The model under review builds one solid part; all positions refer to its coordinate system, in mm. A direction names the side the tool comes from. Coordinates: 2 decimals unless noted, no trailing zeros. Loops run counter-clockwise (first coordinate to the right, second up) from the corner with the lowest first, then second, coordinate; pieces in that order, holes last. Notation, with made-up numbers: M -3,-40 L 39,-40 A19 cw 39,-22 Z; hole C 16.5,45 d3. An arc over 180 degrees is marked long. Use one line per item in the form item = value.
```python
from build123d import *

# Parameters (mm, degrees)
F1_ANGLE = 180
F2_DEPTH = 5.08
F0_W     = 3.2131851465
F0_H     = 5.0839147031
F0_H_2   = 5.0760852969
F0_W_2   = 5.092757754
F0_H_3   = 2.607280938
F3_DEPTH = 5.08


with BuildPart() as f1:
    # F0 (on Front) → F1 (revolve)
    with BuildSketch(Plane.XZ):
        with BuildLine():
            Line((0, 7.1843154948), (0, 9.2163154948))
            Line((0, 9.2163154948), (-5.092757754, 9.2163154948))
            Line((-5.092757754, 9.2163154948), (-12.192, 9.2163154948))
            ThreePointArc((-12.192, 9.2163154948), (-11.524233364, 1.2175235719), (-11.5414183138, -6.8090752834))
            Line((-11.5414183138, -6.8090752834), (-10.7442, -6.8090752834))
            Line((-10.7442, -6.8090752834), (-10.7442, -16.9690752834))
            Line((-10.7442, -16.9690752834), (-12.55264014, -16.9690752834))
            ThreePointArc((-12.55264014, -16.9690752834), (-14.3638496802, -25.8279076884), (-17.018, -34.4716845052))
            Line((-17.018, -34.4716845052), (-14.986, -34.4716845052))
            ThreePointArc((-14.986, -34.4716845052), (-9.9329646545, -13.9500940953), (-10.0076, 7.1843154948))
            Line((-10.0076, 7.1843154948), (0, 7.1843154948))
        make_face()
        with BuildLine():
            Line((-10.7442, -6.8090752834), (-11.5414183138, -6.8090752834))
            ThreePointArc((-11.5414183138, -6.8090752834), (-11.908955512, -11.9028177198), (-12.55264014, -16.9690752834))
            Line((-12.55264014, -16.9690752834), (-10.7442, -16.9690752834))
            Line((-10.7442, -16.9690752834), (-10.7442, -6.8090752834))
        make_face()
    revolve(axis=Axis((0, 0, 8.2003154948), (0, 0, -1)), revolution_arc=F1_ANGLE)

    # F0 (on Front) → F2 (join)
    with BuildSketch(Plane.XZ):
        with BuildLine():
            ThreePointArc((-12.55264014, -16.9690752834), (-11.908955512, -11.9028177198), (-11.5414183138, -6.8090752834))
            Line((-11.5414183138, -6.8090752834), (-12.55264014, -6.8090752834))
            Line((-12.55264014, -6.8090752834), (-12.55264014, -11.8851605803))
            Line((-12.55264014, -11.8851605803), (-12.55264014, -16.9690752834))
        make_face()
        with BuildLine():
            Line((-10.7442, -6.8090752834), (-11.5414183138, -6.8090752834))
            ThreePointArc((-11.5414183138, -6.8090752834), (-11.908955512, -11.9028177198), (-12.55264014, -16.9690752834))
            Line((-12.55264014, -16.9690752834), (-10.7442, -16.9690752834))
            Line((-10.7442, -16.9690752834), (-10.7442, -6.8090752834))
        make_face()
        Polygon((12.55264014, -6.9773710036), (10.7442, -6.9773710036), (10.7442, -17.1373710036), (12.55264014, -17.1373710036), (12.55264014, -12.0534563005), align=None)
    extrude(amount=-F2_DEPTH)

    # F0 (on Front) → F3 (join, symmetric)
    with BuildSketch(Plane.XZ):
        with Locations((14.1592327132, -14.5954136521)):
            Rectangle(F0_W, F0_H)
        with Locations((-14.1592327132, -9.3471179318)):
            Rectangle(F0_W, F0_H_2)
        with Locations((-2.546378877, 10.5199559638)):
            Rectangle(F0_W_2, F0_H_3)
    extrude(amount=F3_DEPTH, both=True)


solid = f1.part
```
1. Add section A-A (y = -2.75). State the section outline as (x, z) points, then the cut area to 3 significant figures.
Response values:
outline = M -15.77,-11.89 L -12.55,-11.89 L -12.55,-6.81 L -15.77,-6.81 Z; M -5.09,9.22 L 0,9.22 L 0,11.82 L -5.09,11.82 Z; M 12.55,-17.14 L 15.77,-17.14 L 15.77,-12.05 L 12.55,-12.05 Z
area = 45.9 mm^2
2. Add section B-B (z = -14). State the section outline as (x, y) points, then the cut area to 3 significant figures.
Response values:
outline = M -12.55,0 L -9.94,0 A9.94 cw 9.94,0 L 12.55,0 L 12.55,-5.08 L 15.77,-5.08 L 15.77,5.08 L 11.03,5.08 A12.14 ccw -11.03,5.08 L -12.55,5.08 Z
area = 117 mm^2
3. Machinability: for faces 5 (the face through (12.553, 3, -10)), 6 (the face through (-13, 5.08, -11)), 7 (the face through (13, 5.08, -13)), 8 (the face through (-3, 5.08, 11)), which of the approach directions +Z, -Z, +X, -X, +Y, -Y give a long, thin tool a straight path to every point of the face, cutting with its end or side? Answer none if there is none.
Response values:
face_5 = +Z, +X, +Y, -Y
face_6 = -X, +Y
face_7 = +X, +Y
face_8 = +Z, +X, -X, +Y
4. The part is to be moulded in two halves that separate along Z. For faces 1 (the face through (-14, 0, -11.885)), 2 (the face through (-12.553, -3, -9)), 3 (the face through (-12.553, 3, -14)), 4 (the face through (14, 0, -12.053)), say which applies: pulls with the +Z half, pulls with the -Z half, needs draft (parallel to the pull), parting line crosses it, or undercut.
Response values:
face_1 = undercut
face_2 = needs draft
face_3 = undercut
face_4 = pulls with the +Z half
5. Insertion check: P1, Ø1.5, axis at x = 3, z = -7.5, coming from the +Y side; P2, Ø1.5, axis at y = 12.5, z = -25.5, coming from the -X side; P3, Ø1, axis at x = 4.5, z = 0, coming from the +Y side; P4, Ø3.5, axis at x = 13.5, y = 0.5, coming from the -Z side. Each pin has a flat end and moves straight along its axis. Give the tip position at first contact, or say it passes through.
Response values:
P1 = 11.36
P2 = -8.17
P3 = 10.76
P4 = -34.47
6. Add section D-D (z = 0.5). State the section outline as (x, y) points, then the cut area to 3 significant figures.
Response values:
outline = M -11.5,0 L -9.42,0 A9.42 cw 9.42,0 L 11.5,0 A11.5 ccw Z
area = 68.2 mm^2
7. Add section C-C (z = -7.5). State the section outline as (x, y) points.
Response values:
outline = M -15.77,-5.08 L -12.55,-5.08 L -12.55,0 L -9.41,0 A9.41 cw 9.41,0 L 12.55,0 L 12.55,5.08 L 10.74,5.08 L 10.74,4.31 A11.57 ccw -10.74,4.31 L -10.74,5.08 L -15.77,5.08 Z
8. Wall thickness on line 1 along Z through (x, y) = (-8.5, 2.25); line 2 along X through (y, z) = (3, -16.5); line 3 along X through (y, z) = (-3.25, -10): over which ranges is each line inside the solid? List them lowest first. Write a range as from..to.
Response values:
line_1 = 7.18..9.22
line_2 = -12.55..-9.83, 9.83..15.77
line_3 = -15.77..-12.55
